from build123d import *

# Parameters (mm, degrees)
ESQUISSE1_W             = 87
ESQUISSE1_H             = 160
ESQUISSE2_R             = 148.5
ENL_V_MAT_EXTRU_1_DEPTH = 12
ESQUISSE2_3_R           = 100
ESQUISSE2_3_R_2         = 90
ENL_V_MAT_EXTRU_2_DEPTH = 53
ESQUISSE4_R             = 90
ENL_V_MAT_EXTRU_3_DEPTH = 56
ESQUISSE10_R            = 60
ENL_V_MAT_EXTRU_4_DEPTH = 56
ENL_V_START             = 3
ESQUISSE11_R            = 65
ENL_V_MAT_EXTRU_7_DEPTH = 13
PER_AGE2_D              = 17
PER_AGE2_DEPTH          = 83
PER_AGE2_CBORE_D        = 25
PER_AGE2_CBORE_DEPTH    = 16


with BuildPart() as part:
    # Esquisse1 → R_volution1 (revolve)
    with BuildSketch(Plane.XY):
        with Locations((43.5, 80)):
            Rectangle(ESQUISSE1_W, ESQUISSE1_H)
    revolve(axis=Axis((87, 0, 0), (-1, 0, 0)))

    # Esquisse2 → Enl_v. mat.-Extru.1 (cut)
    with BuildSketch(Plane(origin=(87, 0, 0), x_dir=(0, 0, -1), z_dir=(1, 0, 0))):
        with Locations(Location((0, 0, 0), (0, 0, 90))):
            Circle(ESQUISSE2_R)
    extrude(amount=-ENL_V_MAT_EXTRU_1_DEPTH, mode=Mode.SUBTRACT)

    # Esquisse2_3 → Enl_v. mat.-Extru.2 (cut)
    with BuildSketch(Plane(origin=(87, 0, 0), x_dir=(0, 0, -1), z_dir=(1, 0, 0))):
        with Locations(Location((0, 0, 0), (0, 0, 90))):
            Circle(ESQUISSE2_3_R)
        with Locations(Location((0, 0, 0), (0, 0, 90))):
            Circle(ESQUISSE2_3_R_2, mode=Mode.SUBTRACT)
    extrude(amount=-ENL_V_MAT_EXTRU_2_DEPTH, mode=Mode.SUBTRACT)

    # Esquisse4 → Enl_v. mat.-Extru.3 (cut)
    with BuildSketch(Plane(origin=(75, 0, 0), x_dir=(0, 0, -1), z_dir=(1, 0, 0))):
        with Locations(Location((0, 0, 0), (0, 0, 90))):
            Circle(ESQUISSE4_R)
    extrude(amount=-ENL_V_MAT_EXTRU_3_DEPTH, mode=Mode.SUBTRACT)

    # Esquisse10 → Enl_v. mat.-Extru.4 (cut)
    with BuildSketch(Plane.ZY):
        with Locations(Location((0, 0, 0), (0, 0, 270))):
            Circle(ESQUISSE10_R)
    extrude(amount=-ENL_V_MAT_EXTRU_4_DEPTH, mode=Mode.SUBTRACT)

    # Esquisse11 → Enl_v. mat.-Extru.7 (cut)
    with BuildSketch(Plane(origin=(0, 0, 0), x_dir=(0, 0, -1), z_dir=(1, 0, 0)).offset(ENL_V_START)):
        with Locations(Location((0, 0, 0), (0, 0, 270))):
            Circle(ESQUISSE11_R)
    extrude(amount=ENL_V_MAT_EXTRU_7_DEPTH, mode=Mode.SUBTRACT)

    # Per_age2
    with Locations(Plane(origin=(0, 130, 0), x_dir=(0, 0, -1), z_dir=(-1, 0, 0))):
        with Locations((0, 0), (0, 260)):
            CounterBoreHole(PER_AGE2_D / 2, PER_AGE2_CBORE_D / 2, PER_AGE2_CBORE_DEPTH, depth=PER_AGE2_DEPTH)


solid = part.part
Work out the finished part from the listing and answer in its coordinate system (mm). A direction names the side the tool comes from. Give positions to 0.01 mm unless a question says otherwise; leave off trailing zeros. Order: outer loops, then holes, each group sorted by start corner. A loop starts at its lowest first (then second) coordinate and runs counter-clockwise, first axis right, second up. Notation, with made-up numbers: M 45,26 L 65,26 A10 ccw 65,36 Z; hole C 78,7.25 d4. An arc over 180 degrees is marked long. Return JSON: item names as keys, results as strings.
Q1. Find the intervals of material crossed by line 1 along Z through (x, y) = (18.3, 0); line 2 along Z through (x, y) = (52, 0); line 3 along X through (y, z) = (-56, -71), in increasing order. Write a range as [from, to].
Answer below:
{"line 1": "z = [-160, -60], [60, 160]", "line 2": "z = [-160, -100], [100, 160]", "line 3": "x = [0, 34]"}
Q2. The mould has two halves that part along Z. Classify faces 5 (the face through (0, 2, 69)), 6 (the face through (44.109, -34.685, 156.195)), 7 (the face through (54.79, 95.38, 30.04)), 8 (the face through (1.48, 59.94, 2.64)): pulls with the +Z half, pulls with the -Z half, needs draft (parallel to the pull), parting line crosses it, or undercut.
Answer below:
{"face 5": "needs draft", "face 6": "parting line crosses it", "face 7": "undercut", "face 8": "undercut"}
Q3. Find section D-D, the plane y = -130. Write down the section's boundary in (x, z), and give its area (3 significant figures).
Answer below:
{"outline": "M 0,-93.27 L 87,-93.27 L 87,-71.78 L 75,-71.78 L 75,-8.5 L 16,-8.5 L 16,-12.5 L 0,-12.5 Z; M 0,12.5 L 16,12.5 L 16,8.5 L 75,8.5 L 75,71.78 L 87,71.78 L 87,93.27 L 0,93.27 Z", "area": "13,100 mm^2"}
Q4. Each of these flat-tipped pins is pushed along its axis until it touches: pin 1 (12 mm diameter, centred on x = 42, y = -13, fed in from -Z); pin 2 (7.5 mm diameter, centred on y = 124, z = -3, fed in from -X); pin 3 (2 mm diameter, centred on x = 24.5, z = 73.5, fed in from +Y); pin 4 (10 mm diameter, centred on y = 130, z = 0, fed in from -X). Where does it stop, or does it pass through?
Answer below:
{"pin 1": "stops at z = -159.85", "pin 2": "stops at x = 16", "pin 3": "stops at y = 142.63", "pin 4": "passes through"}
Q5. Find section C-C, the plane x = 59. Write down the section's boundary in (y, z), and give its area (3 significant figures).
Answer below:
{"outline": "C 0,0 d320; hole C -130,0 d17; hole C 0,0 d200; hole C 130,0 d17", "area": "48,600 mm^2"}
Q6. Find section B-B, the plane z = -20. Write down the section's boundary in (x, y), and give its area (3 significant figures).
Answer below:
{"outline": "M 0,-158.75 L 87,-158.75 L 87,-147.15 L 75,-147.15 L 75,-97.98 L 34,-97.98 L 34,-87.75 L 19,-87.75 L 19,-56.57 L 16,-56.57 L 16,-61.85 L 3,-61.85 L 3,-56.57 L 0,-56.57 Z; M 0,56.57 L 3,56.57 L 3,61.85 L 16,61.85 L 16,56.57 L 19,56.57 L 19,87.75 L 34,87.75 L 34,97.98 L 75,97.98 L 75,147.15 L 87,147.15 L 87,158.75 L 0,158.75 Z", "area": "11,100 mm^2"}
Q7. Which of the six approach directions +Z, -Z, +X, -X, +Y, -Y give full straight-line access (tool end or side, diameter ignored) to faces 1 (the face through (16, -19, 57.5)), 2 (the face through (7.888, 117.606, 1.627)), 3 (the face through (87, -46.7, 141.5)), 4 (the face through (26.605, 83.137, -34.471))?
Answer below:
{"face 1": "none", "face 2": "-X", "face 3": "+Z, -Z, +X, +Y, -Y", "face 4": "+X"}
Q8. Find section A-A, the plane y = 0. Write down the section's boundary in (x, z), and give its area (3 significant figures).
Answer below:
{"outline": "M 0,-160 L 87,-160 L 87,-148.5 L 75,-148.5 L 75,-100 L 34,-100 L 34,-90 L 19,-90 L 19,-60 L 16,-60 L 16,-65 L 3,-65 L 3,-60 L 0,-60 Z; M 0,60 L 3,60 L 3,65 L 16,65 L 16,60 L 19,60 L 19,90 L 34,90 L 34,100 L 75,100 L 75,148.5 L 87,148.5 L 87,160 L 0,160 Z", "area": "11,000 mm^2"}
